```python
from build123d import *

# Parameters (mm, degrees)
CUT_EXTRUDE_1_DEPTH      = 192.562000407
CUT_EXTRUDE_1_DEPTH_BACK = 192.562000407
SKETCH_2_W               = 15
SKETCH_2_H               = 2
SKETCH_3_R               = 2.25
CUT_EXTRUDE_2_DEPTH      = 10


with BuildPart() as part:
    # 草圖1 → 旋轉1 (revolve)
    with BuildSketch(Plane.XY, mode=Mode.PRIVATE) as revolve_1_sk:
        with BuildLine():
            Line((-188, 0), (-188, 6))
            Line((-188, 6), (-166, 6))
            Line((-166, 6), (-166, 16))
            Line((-166, 16), (-163, 16))
            Line((-163, 16), (-163, 26))
            Line((-163, 26), (-79, 26))
            Line((-79, 26), (-79, 21))
            ThreePointArc((-79, 21), (-77.535533906, 24.535533906), (-74, 26))
            Line((-74, 26), (-10, 26))
            Line((-10, 26), (-10, 13))
            Line((-10, 13), (0, 13))
            Line((0, 13), (0, 0))
            Line((0, 0), (-188, 0))
        make_face()
    revolve(revolve_1_sk.sketch.rotate(Axis((-188, 0, 0), (1, 0, 0)), 90), axis=Axis((-188, 0, 0), (1, 0, 0)))

    # 草圖2 → 伸長1 (cut, two sides: drawn at the far end of the back side and taken through both)
    with BuildSketch(Plane.XY.offset(-CUT_EXTRUDE_1_DEPTH_BACK)):
        with Locations((-180.5, 5)):
            Rectangle(SKETCH_2_W, SKETCH_2_H)
    extrude(amount=CUT_EXTRUDE_1_DEPTH + CUT_EXTRUDE_1_DEPTH_BACK, mode=Mode.SUBTRACT)

    # 草圖3 → 伸長2 (cut)
    with BuildSketch(Plane.ZY.offset(166)):
        with Locations((0, 20)):
            Circle(SKETCH_3_R)
        with Locations((20, 0)):
            Circle(SKETCH_3_R)
        with Locations((0, -20)):
            Circle(SKETCH_3_R)
        with Locations((-20, 0)):
            Circle(SKETCH_3_R)
    extrude(amount=-CUT_EXTRUDE_2_DEPTH, mode=Mode.SUBTRACT)


solid = part.part
```
Build history of the part. All positions in model axes, mm. A direction names the side the tool comes from. Round coordinates to 2 decimals unless told otherwise and drop trailing zeros. Loops run counter-clockwise (first coordinate to the right, second up) from the corner with the lowest first, then second, coordinate; pieces in that order, holes last. Notation, with made-up numbers: M 65.25,33.5 L 100.25,33.5 A18 cw 100.25,57.5 Z; hole C 76,29 d9. An arc over 180 degrees is marked long. Answer as CSV lines item,"result".
1. Cut at C-C on x = -41. Write the cut outline in (y, z).
Resolved:
outline,"C 0,0 d52"
2. Flat gauge pins, fed straight in: P1, Ø5, axis at y = 20, z = 0, coming from the +X side; P2, Ø6, axis at x = -20, y = 12, coming from the +Z side; P3, Ø2, axis at y = -20, z = -1, coming from the -X side. Where does each tip first touch, or does it go through?
Resolved:
P1,"stops at x = -10"
P2,"stops at z = 24.39"
P3,"stops at x = -156"
3. Wall check: probe 1 along Y at (x, z) = (-160.75, 0); probe 2 along X at (y, z) = (10.5, 6); probe 3 along X at (y, z) = (10, 13.5). Give the ranges that are in metal, low to high. Write a range as [from, to].
Resolved:
probe 1,"y = [-26, -22.25], [-17.75, 17.75], [22.25, 26]"
probe 2,"x = [-166, 0]"
probe 3,"x = [-163, -10]"
4. 3-axis set-ups, long thin cutter, end or side, ignore diameter. For faces 1 (the cylindrical face through (-4.93, 7.91, -10.316)), 2 (the flat face through (-188, -1, 0)), 3 (the cylindrical face through (-164.48, 15.62, -3.47)), 4 (the flat face through (-181, 4, 0)), 5 (the cylindrical face through (-41.552, 15.821, -20.633)): which of +Z, -Z, +X, -X, +Y, -Y reach the whole face in a straight line?
Resolved:
face 1,"+X"
face 2,"+Z, -Z, -X, +Y, -Y"
face 3,"-X"
face 4,"+Z, -Z, -X, +Y"
face 5,"+X, -X"
5. Cut at D-D on x = -175.5. Write the cut outline in (y, z).
Resolved:
outline,"M 4,-4.47 L 4,4.47 A6 ccw long Z"
